```python
from build123d import *

# Parameters (mm, degrees)
SKETCH4_W          = 13.208
SKETCH4_H          = 36.83
SKETCH4_W_2        = 19.304
CUT_EXTRUDE1_DEPTH = 7.62


with BuildPart() as part:
    # Sketch1 → Loft1 section 0
    with BuildSketch(Plane(origin=(0, 0, 0), x_dir=(1, 0, 0), z_dir=(0, 1, 0))):
        with BuildLine():
            Line((0, 7.112), (6.35, 7.112))
            Line((6.35, 7.112), (6.35, 35.052))
            Line((6.35, 35.052), (0, 35.052))
            Line((0, 35.052), (0, 42.164))
            Line((0, 42.164), (6.35, 42.164))
            Line((6.35, 42.164), (6.35, 45.974))
            Line((6.35, 45.974), (84.074, 45.974))
            Line((84.074, 45.974), (84.074, 42.164))
            Line((84.074, 42.164), (90.424, 42.164))
            Line((90.424, 42.164), (90.424, 35.052))
            Line((90.424, 35.052), (84.074, 35.052))
            Line((84.074, 35.052), (84.074, 7.112))
            Line((84.074, 7.112), (90.424, 7.112))
            Line((90.424, 7.112), (90.424, 0))
            Line((90.424, 0), (84.074, 0))
            Line((84.074, 0), (84.074, -3.81))
            Line((84.074, -3.81), (6.35, -3.81))
            Line((6.35, -3.81), (6.35, 0))
            Line((6.35, 0), (0, 0))
            Line((0, 0), (0, 7.112))
        make_face()
    # Sketch2 → Loft1 section 1
    with BuildSketch(Plane(origin=(0, 2.7667966, 0), x_dir=(1, 0, 0), z_dir=(0, 1, 0))):
        with BuildLine():
            Line((90.424, -0.3888486), (90.424, 6.7231514))
            Line((90.424, 6.7231514), (84.074, 6.7231514))
            Line((84.074, 6.7231514), (84.074, 34.6631514))
            Line((84.074, 34.6631514), (90.424, 34.6631514))
            Line((90.424, 34.6631514), (90.424, 41.7751514))
            Line((90.424, 41.7751514), (84.074, 41.7751514))
            Line((84.074, 41.7751514), (84.074, 45.5851514))
            Line((84.074, 45.5851514), (6.35, 45.5851514))
            Line((6.35, 45.5851514), (6.35, 41.7751514))
            Line((6.35, 41.7751514), (0, 41.7751514))
            Line((0, 41.7751514), (0, 34.6631514))
            Line((0, 34.6631514), (6.35, 34.6631514))
            Line((6.35, 34.6631514), (6.35, 6.7231514))
            Line((6.35, 6.7231514), (0, 6.7231514))
            Line((0, 6.7231514), (0, -0.3888486))
            Line((0, -0.3888486), (6.35, -0.3888486))
            Line((6.35, -0.3888486), (6.35, -4.1988486))
            Line((6.35, -4.1988486), (84.074, -4.1988486))
            Line((84.074, -4.1988486), (84.074, -0.3888486))
            Line((84.074, -0.3888486), (90.424, -0.3888486))
        make_face()
    loft()

    # Sketch4 → Cut-Extrude1 (cut)
    with BuildSketch(Plane(origin=(0, 2.7667966, 0), x_dir=(1, 0, 0), z_dir=(0, 1, 0))):
        with Locations((45.212, 21.082)):
            Rectangle(SKETCH4_W, SKETCH4_H)
        with Locations((22.479, 21.082)):
            Rectangle(SKETCH4_W_2, SKETCH4_H)
        with Locations((67.945, 21.082)):
            Rectangle(SKETCH4_W_2, SKETCH4_H)
    extrude(amount=-CUT_EXTRUDE1_DEPTH, mode=Mode.SUBTRACT)


solid = part.part
```
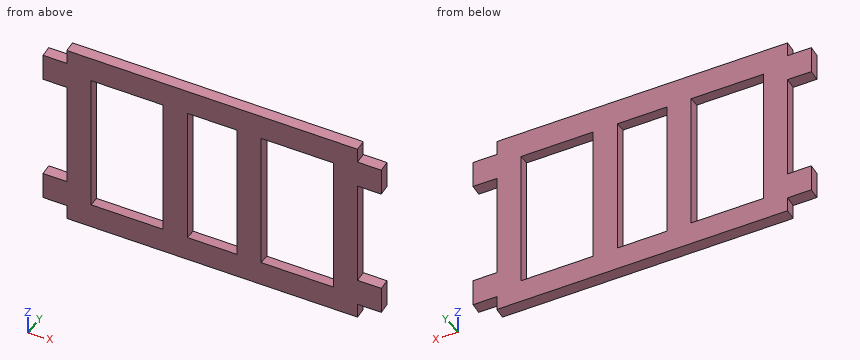
CAD build for the part. Positions are in the model's coordinates, mm. Round coordinates to 2 decimals unless told otherwise and drop trailing zeros. Loops run counter-clockwise (first coordinate to the right, second up) from the corner with the lowest first, then second, coordinate; pieces in that order, holes last. Notation, with made-up numbers: M 5,29.5 L 64,29.5 A29 ccw 64,61.5 Z; hole C 18,79 d11. An arc over 180 degrees is marked long. Return JSON: item names as keys, results as strings. Group by question number.
(1) Saw through at A-A, the plane x = 44. List the corners of the cut face in (y, z), and give its area (3 significant figures).
(2) Wall check: probe 1 along X at (y, z) = (0.3, -29.5); probe 2 along X at (y, z) = (1.9, -3); probe 3 along X at (y, z) = (0.45, -43.5). Give the ranges that are in metal, low to high. Write a range as [from, to].
(3) Drop flat-ended pins along their axis: P1, Ø1.4, axis at y = 1, z = -27.5, coming from the -X side; P2, Ø1.4, axis at x = 20.5, y = 1.5, coming from the +Z side; P3, Ø1.5, axis at x = 42, y = 0.5, coming from the +Z side. Give the stop position or say it passes through.
(4) Saw through at B-B, the plane z = -4. Give the number of separate pieces and of enclosed holes in the cut face, and give its area (3 significant figures).
Answer list:
{
 "1": {"outline": "M 0,-45.97 L 2.77,-45.59 L 2.77,-39.5 L 0,-39.5 Z; M 0,-2.67 L 2.77,-2.67 L 2.77,4.2 L 0,3.81 Z", "area": "35.8 mm2"},
 "2": {"probe 1": "[6.35, 12.83], [32.13, 38.61], [51.82, 58.29], [77.6, 84.07]", "probe 2": "[0, 12.83], [32.13, 38.61], [51.82, 58.29], [77.6, 90.42]", "probe 3": "[6.35, 84.07]"},
 "3": {"P1": "x = 6.35", "P2": "z = 4.12", "P3": "z = 3.99"},
 "4": {"separate pieces": "4", "enclosed holes": "0", "area": "107 mm2"}
}
